```python
from build123d import *

# Parameters (mm, degrees)
SKETCH_1_W      = 80
SKETCH_1_H      = 35
SKETCH_1_R      = 4.25
EXTRUDE_1_DEPTH = 2.5
FILLET_1_R      = 1


with BuildPart() as part:
    # Эскиз1 → Бобышка-Вытянуть1 (new body)
    with BuildSketch(Plane.XY):
        Rectangle(SKETCH_1_W, SKETCH_1_H)
        with Locations((-26, 0)):
            Circle(SKETCH_1_R, mode=Mode.SUBTRACT)
        with Locations((26, 0)):
            Circle(SKETCH_1_R, mode=Mode.SUBTRACT)
    extrude(amount=EXTRUDE_1_DEPTH)

    # Скругление1
    fillet_1_edges = [part.edges().sort_by_distance(p)[0] for p in [
        (40, -17.5, 1.25),
        (-40, -17.5, 1.25),
        (-40, 17.5, 1.25),
        (40, 17.5, 1.25),
    ]]
    fillet(fillet_1_edges, radius=FILLET_1_R)


solid = part.part
```
Could you check a few things on this model? Use its own coordinates, in mm. Round coordinates to 2 decimals unless told otherwise and drop trailing zeros. Loops run counter-clockwise (first coordinate to the right, second up) from the corner with the lowest first, then second, coordinate; pieces in that order, holes last. Notation, with made-up numbers: (-14.5, -35.75) - (26.5, -35.75) arc R20 ccw to (26.5, 0.25) - close; hole circle Ø3 at (-7.5, -9.75). An arc over 180 degrees is marked (long way). Answer in a Markdown table with one row per item. Add a question column.
(1) If we mould it in two halves opening along Y, with no side actions, what happens to faces 1 (the face through (-1, 0, 0)), 2 (the face through (-1, -17.5, 1)), 3 (the face through (22.868, 2.872, 1.232)), 4 (the face through (-30.246, 0.187, 1.232))? For each: pulls with the +Y half, pulls with the -Y half, needs draft (parallel to the pull), parting line crosses it, or undercut.
(2) I need wall thicknesses on line 1 along Y through (x, z) = (26, 1.3); line 2 along Y through (x, z) = (-23.5, 0.55). Which ranges of each line are inside material? Lowest first, please.
(3) If we section it at C-C (z = 1.65): Please give me the cut outline in (x, y).
(4) If we section it at B-B (y = 0): Please give me the cut outline in (x, z), plus the area to 4 significant figures.
(5) If we section it at A-A (x = 26): Please give me the cut outline in (y, z), plus the area to 4 significant figures.
Model answer:
| question | item | result |
|---|---|---|
| 1 | face 1 | needs draft |
| 1 | face 2 | pulls with the -Y half |
| 1 | face 3 | undercut |
| 1 | face 4 | undercut |
| 2 | line 1 | y = -17.5 to -4.25, 4.25 to 17.5 |
| 2 | line 2 | y = -17.5 to -3.44, 3.44 to 17.5 |
| 3 | outline | (-40, -16.5) arc R1 ccw to (-39, -17.5) - (39, -17.5) arc R1 ccw to (40, -16.5) - (40, 16.5) arc R1 ccw to (39, 17.5) - (-39, 17.5) arc R1 ccw to (-40, 16.5) - close; hole circle Ø8.5 at (-26, 0); hole circle Ø8.5 at (26, 0) |
| 4 | outline | (-40, 0) - (-30.25, 0) - (-30.25, 2.5) - (-40, 2.5) - close; (-21.75, 0) - (21.75, 0) - (21.75, 2.5) - (-21.75, 2.5) - close; (30.25, 0) - (40, 0) - (40, 2.5) - (30.25, 2.5) - close |
| 4 | area | 157.5 mm² |
| 5 | outline | (-17.5, 0) - (-4.25, 0) - (-4.25, 2.5) - (-17.5, 2.5) - close; (4.25, 0) - (17.5, 0) - (17.5, 2.5) - (4.25, 2.5) - close |
| 5 | area | 66.25 mm² |
